The listing builds one solid part. Answer for the finished solid, in the listing's coordinates (mm). Face numbers are marked on the shaded views. A direction names the side the tool comes from. Round coordinates to 2 decimals unless told otherwise and drop trailing zeros. Write each loop counter-clockwise with the first axis right and the second up, starting at its lowest first coordinate (ties: lowest second). Pieces come first, ordered by that corner, then holes. Notation, with made-up numbers: (12, 27) - (43, 27) arc R16 cw to (43, 31) - close; hole circle Ø6 at (-28, 38.5). An arc over 180 degrees is marked (long way). Answer in a Markdown table with one row per item.
Autodesk Inventor part; units mm, degrees
ref_plane "YZ Plane" through (0, 0, 0) normal (1, 0, 0) x (0, 1, 0)
ref_plane "XZ Plane" through (0, 0, 0) normal (0, 1, 0) x (-1, 0, 0)
ref_plane "XY Plane" through (0, 0, 0) normal (0, 0, 1) x (1, 0, 0)
sketch "Skizze1" plane through (0, 0, 0) normal (0, 0, 1) x (1, 0, 0)
  line L0 (-9.8, 0) -> (9.8, 0)
  line L1 (0, -2) -> (0, 12)
  line L2 (-7, 0) -> (7, 0)
  line L3 (7, 0) -> (7, 10)
  line L4 (-7, 10) -> (-7, 0)
  line L5 (3.5, 10) -> (3.5, 5)
  line L6 (3.5, 5) -> (-3.5, 5)
  line L7 (-3.5, 5) -> (-3.5, 10)
  line L8 (7, 10) -> (3.5, 10)
  line L9 (-3.5, 10) -> (-7, 10)
  point P0 (0, 0)
  dimension "d0" = 10
  dimension "d1" = 5
  dimension "d3" = 3.5
  dimension "d6" = 7
extrude "Extrusion1" add sketch "Skizze1" along normal blind 15
sketch "Skizze2" plane through (7, 0, 0) normal (1, 0, 0) x (0, 0, -1)
  line L0 (-15, 10) -> (-15, 0)
  line L1 (0, 0) -> (-15, 0)
  line L2 (0, 0) -> (0, 10)
  line L3 (-15, 5) -> (0, 5)
  point P0 (-11, 5)
  point P1 (-4, 5)
  dimension "d9" = 4
  dimension "d10" = 4
  dimension "d11" = 5
hole "Bohrung1" at (7, 5, 11) at (7, 5, 4) direction (-1, 0, 0) diameter 2.459 end through all
properties part number "13_0204_052"
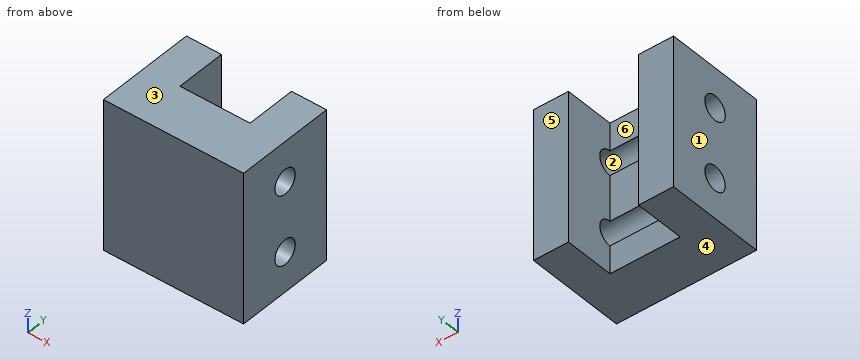
(1) Section B-B (z = 4) is taken. Give the vertices of the cut face in (x, y).
Checked values:
| item | result |
|---|---|
| outline | (-7, 0) - (7, 0) - (7, 3.77) - (-7, 3.77) - close; (-7, 6.23) - (-3.5, 6.23) - (-3.5, 10) - (-7, 10) - close; (3.5, 6.23) - (7, 6.23) - (7, 10) - (3.5, 10) - close |
(2) Section D-D (x = 5.75) is taken. Give the vertices of the cut face in (y, z).
Checked values:
| item | result |
|---|---|
| outline | (0, 0) - (10, 0) - (10, 15) - (0, 15) - close; hole circle Ø2.46 at (5, 4); hole circle Ø2.46 at (5, 11) |
(3) Section C-C (x = 0.5) is taken. Give the vertices of the cut face in (y, z), and give its area (3 significant figures).
Checked values:
| item | result |
|---|---|
| outline | (0, 0) - (5, 0) - (5, 2.77) arc R1.23 cw to (5, 5.23) - (5, 9.77) arc R1.23 cw to (5, 12.23) - (5, 15) - (0, 15) - close |
| area | 70.3 mm2 |
(4) For a pull along Z with two mould halves and no side action, classify the marked faces 1, 2, 3 and 4 as pulls with the +Z half, pulls with the -Z half, needs draft (parallel to the pull), parting line crosses it, or undercut.
Checked values:
| item | result |
|---|---|
| face 1 | needs draft |
| face 2 | undercut |
| face 3 | pulls with the +Z half |
| face 4 | pulls with the -Z half |
(5) For the marked faces 5 and 6, determine the directions among +Z, -Z, +X, -X, +Y, -Y from which every point of the face is accessible in a straight line to the end or side of a thin tool.
Checked values:
| item | result |
|---|---|
| face 5 | +Z, -Z, +X, -X, +Y |
| face 6 | +Z, -Z, +Y |
(6) Flat-ended cylindrical pins translate along their axes: pin 1 (0.8 mm diameter, centred on x = -0.5, z = 1.5, fed in from +Y); pin 2 (5 mm diameter, centred on x = -2.5, y = 8, fed in from -Z); pin 3 (2 mm diameter, centred on y = 5, z = 4, fed in from -X). Find the tip coordinate at first contact, or state that the pin passes through.
Checked values:
| item | result |
|---|---|
| pin 1 | stops at y = 5 |
| pin 2 | stops at z = 0 |
| pin 3 | passes through |
(7) Find the intervals of material crossed by line 1 (Z direction, x = -3.75, y = 5); line 2 (X direction, y = 9, z = 9.5); line 3 (Z direction, x = -6.5, y = 4.5), in increasing order.
Checked values:
| item | result |
|---|---|
| line 1 | z = 0 to 2.77, 5.23 to 9.77, 12.23 to 15 |
| line 2 | x = -7 to -3.5, 3.5 to 7 |
| line 3 | z = 0 to 2.88, 5.12 to 9.88, 12.12 to 15 |
(8) Section A-A (y = 9.25) is taken. Give the vertices of the cut face in (x, z).
Checked values:
| item | result |
|---|---|
| outline | (-7, 0) - (-3.5, 0) - (-3.5, 15) - (-7, 15) - close; (3.5, 0) - (7, 0) - (7, 15) - (3.5, 15) - close |
